Autodesk Inventor part; units mm, degrees
ref_plane "Начальная плоскость" through (0, 0, 0) normal (0, 0, 1) x (1, 0, 0)
ref_plane "Конечная плоскость" through (0, 0, 1800) normal (0, 0, 1) x (1, 0, 0)
ref_plane "YZ Plane" through (0, 0, 0) normal (1, 0, 0) x (0, 1, 0)
ref_plane "Начальная плоскость" through (0, 0, 0) normal (0, 0, 1) x (1, 0, 0)
ref_plane "Конечная плоскость" through (0, 0, 1800) normal (0, 0, 1) x (1, 0, 0)
sketch "Sketch2" plane through (0, 0, 0) normal (0, 0, 1) x (1, 0, 0)
  line L0 (-4.4, -5) -> (-4.4, 22)
  line L1 (-6.4, 22) -> (-4.4, 22)
  line L2 (-6.4, -5) -> (-6.4, 22)
  line L3 (-1.4, -10) -> (18.6, -10)
  line L4 (18.6, -8) -> (18.6, -10)
  line L5 (-1.4, -8) -> (18.6, -8)
  arc A0 (-4.4, -5) -> (-1.4, -8) centre (-1.4, -5) ccw
  arc A1 (-6.4, -5) -> (-1.4, -10) centre (-1.4, -5) ccw
  line L6 (0, 30.2071) -> (0, -6.2426) construction
  line L7 (-5.2426, 0) -> (24.2071, 0) construction
  point P0 (-4.4, -8)
  point P1 (-6.4, -10)
  dimension "d4" = 25
  dimension "d6" = 32
  dimension "d8" = 2
  dimension "d10" = 2
  dimension "d17" = 3
  dimension "d18" = 5
  dimension "d21" = 6.4
  dimension "d22" = 10
extrude "Базовый элемент" add sketch "Sketch2" along normal up to surface (1800 mm away) from surface at 0
sketch "Sketch3" plane through (0, 0, 0) normal (0, 0, 1) x (1, 0, 0)
  line L0 (0, 0) -> (10, 0)
ref_plane "Work Plane10" through (0, 0, 0) normal (0, -1, 0) x (1, 0, 0)
sketch "Sketch4" plane through (0, 0, 0) normal (0, -1, 0) x (1, 0, 0)
  line L0 (-2, 0) -> (12, 0)
  line L1 (-2, 1800) -> (12, 1800)
  dimension "d24" = 1800
equation "\"d8\" = ParT"
equation "\"d10\" = ParT"
equation "\"d17\" = R"
equation "\"d18\" = R + ParT"
equation "\"d21\" = ex"
equation "\"d22\" = ey"
equation "\"d11\" = G_L"
equation "\"b\" = 32"
equation "\"ParT\" = 2"
equation "\"R\" = 3"
equation "\"G_L\" = d24"
equation "\"a\" = 25"
equation "\"G_OFFSET_START\" = 0"
equation "\"G_OFFSET_END\" = 0"
equation "\"ex\" = 6.4"
equation "\"ey\" = 10"
properties part number "Угол 32x25x2-1800 ГОСТ 19772-93" material "Сталь, мягкая"
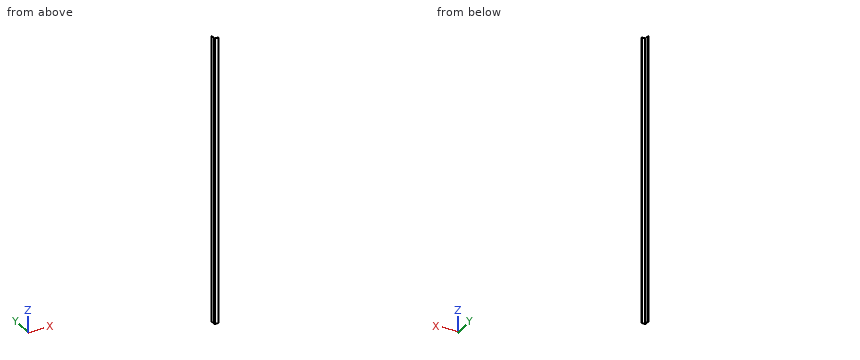
Here's how the part is built. I have some questions about the finished solid (model axes, mm). Coordinates: 2 decimals unless noted, no trailing zeros. Loops run counter-clockwise (first coordinate to the right, second up) from the corner with the lowest first, then second, coordinate; pieces in that order, holes last. Notation, with made-up numbers: (50.5, -18.75) -> (78.5, -18.75) arc R10 ccw to (78.5, -9.75) -> close; hole circle Ø6 at (25, 26.25). An arc over 180 degrees is marked (long way). Use one line per item in the form item = value. Start each with the question number.
(1) Please list where these lines run through material, in increasing order: line 1 along Y through (x, z) = (-2.5, 1135); line 2 along X through (y, z) = (-9, 1115.5); line 3 along Y through (x, z) = (4, 1408).
(2) If we section it at A-A (z = 392.5): Please give me the cut outline in (x, y), then the cut area to 3 significant figures.
(3) If we section it at B-B (y = 12.5): Please give me the cut outline in (x, z), then the cut area to 3 significant figures.
(4) Will these pins go through, and if not, where does the flat tip stop? pin 1 (6 mm diameter, centred on x = -2, y = 15, fed in from -Z); pin 2 (3 mm diameter, centred on x = 9, z = 1288, fed in from +Y); pin 3 (8 mm diameter, centred on y = 13, z = 526.5, fed in from +X); pin 4 (10 mm diameter, centred on x = 2, y = -0.5, fed in from +Z).
(5) If we section it at C-C (x = 13): Please give me the cut outline in (y, z).
Verdict:
q1.line_1 = -9.88 to -7.79
q1.line_2 = -4.4 to 18.6
q1.line_3 = -10 to -8
q2.outline = (-6.4, -5) arc R5 ccw to (-1.4, -10) -> (18.6, -10) -> (18.6, -8) -> (-1.4, -8) arc R3 cw to (-4.4, -5) -> (-4.4, 22) -> (-6.4, 22) -> close
q2.area = 107 mm²
q3.outline = (-6.4, 0) -> (-4.4, 0) -> (-4.4, 1800) -> (-6.4, 1800) -> close
q3.area = 3,600 mm²
q4.pin_1 = 0
q4.pin_2 = -8
q4.pin_3 = -4.4
q4.pin_4 = through
q5.outline = (-10, 0) -> (-8, 0) -> (-8, 1800) -> (-10, 1800) -> close
